CAD build for the part. Positions are in the model's coordinates, mm. Give positions to 0.01 mm unless a question says otherwise; leave off trailing zeros. Write each loop counter-clockwise with the first axis right and the second up, starting at its lowest first coordinate (ties: lowest second). Pieces come first, ordered by that corner, then holes. Notation, with made-up numbers: (25.5, 69.25) -> (53.5, 69.25) arc R20 cw to (53.5, 90.25) -> close; hole circle Ø4 at (88.5, -39). An arc over 180 degrees is marked (long way). Use one line per item in the form item = value. Start each with the question number.
from build123d import *

# Parameters (mm, degrees)
PAD017_DEPTH    = 1
PAD018_DEPTH    = 2
SKETCH041_R     = 3.5
PAD019_DEPTH    = 3.3
SKETCH042_R     = 2.55
POCKET018_DEPTH = 4.3
SKETCH043_R     = 2.8
PAD020_DEPTH    = 1.5
SKETCH044_R     = 2.1
POCKET019_DEPTH = 3
SKETCH045_R     = 3.5
PAD021_DEPTH    = 5.8
SKETCH046_R     = 2.55
POCKET020_DEPTH = 3.8
SKETCH047_R     = 2.6
POCKET021_DEPTH = 1.7
POCKET025_DEPTH = 2


with BuildPart() as part:
    # Sketch038 → Pad017 (new body)
    with BuildSketch(Plane.XZ):
        with BuildLine():
            ThreePointArc((6, 16), (8.928932, 8.928932), (16, 6))
            Line((16, 6), (185.51, 6))
            ThreePointArc((185.51, 6), (192.581068, 8.928932), (195.51, 16))
            Line((195.51, 16), (195.51, 107.04))
            ThreePointArc((195.51, 107.04), (192.581068, 114.111068), (185.51, 117.04))
            Line((185.51, 117.04), (96.718237, 117.04))
            ThreePointArc((96.718237, 117.04), (95.677689, 117.177713), (94.70879, 117.58137))
            Line((94.70879, 117.58137), (67.290497, 133.511257))
            ThreePointArc((67.290497, 133.511257), (65.837149, 134.116742), (64.276328, 134.323311))
            Line((64.276328, 134.323311), (41.441667, 134.323311))
            ThreePointArc((41.441667, 134.323311), (36.445319, 132.985672), (32.785632, 129.330611))
            Line((32.785632, 129.330611), (9.11531, 88.412125))
            ThreePointArc((9.11531, 88.412125), (6.792371, 82.814067), (6, 76.805203))
            Line((6, 76.805203), (6, 16))
        make_face()
    extrude(amount=PAD017_DEPTH)

    # Sketch040 (on Face15 of Pad017) → Pad018 (join)
    with BuildSketch(Plane(origin=(0, 0, 0), x_dir=(1, 0, 0), z_dir=(0, 1, 0))):
        with BuildLine():
            Line((16.1, -9.1), (185.41, -9.1))
            ThreePointArc((192.41, -16.1), (190.359747, -11.150253), (185.41, -9.1))
            Line((192.41, -16.1), (192.41, -106.94))
            ThreePointArc((185.41, -113.94), (190.359747, -111.889747), (192.41, -106.94))
            Line((185.41, -113.94), (95.883059, -113.94))
            ThreePointArc((95.883059, -113.94), (94.842511, -114.077713), (93.873612, -114.48137))
            Line((93.873612, -114.48137), (66.455319, -130.411257))
            ThreePointArc((63.44115, -131.223311), (65.001971, -131.016742), (66.455319, -130.411257))
            Line((63.44115, -131.223311), (41.499346, -131.223311))
            ThreePointArc((35.440122, -127.728421), (38.001902, -130.286964), (41.499346, -131.223311))
            Line((35.440122, -127.728421), (12.21531, -87.580081))
            ThreePointArc((9.1, -75.97316), (9.892371, -81.982024), (12.21531, -87.580081))
            Line((9.1, -75.97316), (9.1, -16.1))
            ThreePointArc((16.1, -9.1), (11.150253, -11.150253), (9.1, -16.1))
        make_face()
    extrude(amount=PAD018_DEPTH)

    # Sketch041 (on Face31 of Pad018) → Pad019 (join)
    with BuildSketch(Plane(origin=(0, 2, 0), x_dir=(1, 0, 0), z_dir=(0, 1, 0))):
        with Locations((145.11, -12.99)):
            Circle(SKETCH041_R)
        with Locations((64.452126, -127.45504)):
            Circle(SKETCH041_R)
        with Locations((14.14, -13.51)):
            Circle(SKETCH041_R)
        with Locations((19.14, -90.503884)):
            Circle(SKETCH041_R)
        with Locations((105.9, -108.54)):
            Circle(SKETCH041_R)
        with Locations((74.12, -12.75)):
            Circle(SKETCH041_R)
    extrude(amount=PAD019_DEPTH)

    # Sketch042 (on Face38 of Pad019) → Pocket018 (cut)
    with BuildSketch(Plane(origin=(0, 5.3, 0), x_dir=(1, 0, 0), z_dir=(0, 1, 0))):
        with Locations((145.11, -12.99)):
            Circle(SKETCH042_R)
        with Locations((19.14, -90.503884)):
            Circle(SKETCH042_R)
        with Locations((64.452126, -127.45504)):
            Circle(SKETCH042_R)
        with Locations((105.9, -108.54)):
            Circle(SKETCH042_R)
        with Locations((14.14, -13.51)):
            Circle(SKETCH042_R)
        with Locations((74.12, -12.75)):
            Circle(SKETCH042_R)
    extrude(amount=-POCKET018_DEPTH, mode=Mode.SUBTRACT)

    # Sketch043 (on Face31 of Pocket018) → Pad020 (join)
    with BuildSketch(Plane(origin=(0, 2, 0), x_dir=(1, 0, 0), z_dir=(0, 1, 0))):
        with Locations((185.580566, -111.078545)):
            Circle(SKETCH043_R)
    extrude(amount=PAD020_DEPTH)

    # Sketch044 (on Face45 of Pad020) → Pocket019 (cut)
    with BuildSketch(Plane(origin=(0, 3.5, 0), x_dir=(1, 0, 0), z_dir=(0, 1, 0))):
        with Locations((185.580566, -111.078545)):
            Circle(SKETCH044_R)
    extrude(amount=-POCKET019_DEPTH, mode=Mode.SUBTRACT)

    # Sketch045 (on Face31 of Pocket019) → Pad021 (join)
    with BuildSketch(Plane(origin=(0, 2, 0), x_dir=(1, 0, 0), z_dir=(0, 1, 0))):
        with Locations((188.21, -14.18)):
            Circle(SKETCH045_R)
    extrude(amount=PAD021_DEPTH)

    # Sketch046 (on Face45 of Pad021) → Pocket020 (cut)
    with BuildSketch(Plane(origin=(0, 7.8, 0), x_dir=(1, 0, 0), z_dir=(0, 1, 0))):
        with Locations((188.21, -14.18)):
            Circle(SKETCH046_R)
    extrude(amount=-POCKET020_DEPTH, mode=Mode.SUBTRACT)

    # Sketch047 (on Face5 of Pocket020) → Pocket021 (cut)
    with BuildSketch(Plane.XZ.offset(1)):
        with Locations((187.41, 103.94)):
            Circle(SKETCH047_R)
        with Locations((40.34577, 126.223311)):
            Circle(SKETCH047_R)
        with Locations((14.1, 77.580081)):
            Circle(SKETCH047_R)
        with Locations((103.873612, 14.1)):
            Circle(SKETCH047_R)
        with Locations((187.41, 19.1)):
            Circle(SKETCH047_R)
        with Locations((120.883059, 108.94)):
            Circle(SKETCH047_R)
        with Locations((19.1, 14.1)):
            Circle(SKETCH047_R)
    extrude(amount=-POCKET021_DEPTH, mode=Mode.SUBTRACT)

    # Sketch056 (on Face38 of Pocket021) → Pocket025 (cut)
    with BuildSketch(Plane(origin=(0, 2, 0), x_dir=(1, 0, 0), z_dir=(0, 1, 0))):
        Polygon((146.906174, -8.786863), (146.906174, -9.81445), (150.102356, -9.81445), (150.102356, -15.780038), (161.659576, -15.780038), (161.659576, -9.891122), (164.762894, -9.891122), (164.762894, -8.786863), align=None)
    extrude(amount=-POCKET025_DEPTH, mode=Mode.SUBTRACT)


with BuildPart() as part_1:
    # Body004 placement: moved
    add(part.part.moved(Location((0, -118.5, 0))))


solid = part_1.part
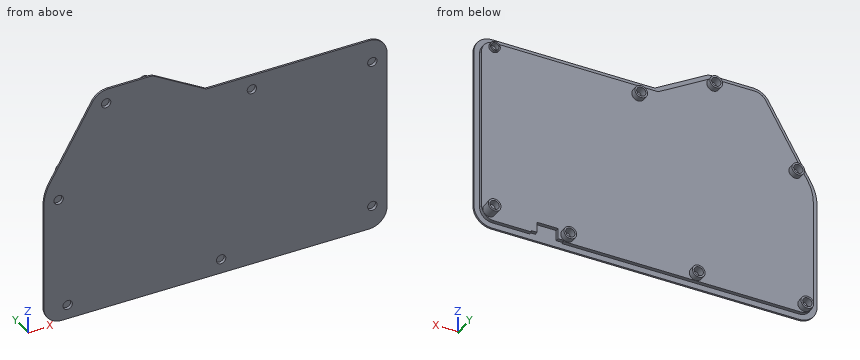
1) Pin check, flat tips, straight feed: pin 1 (4 mm diameter, centred on x = 102.5, z = 14, fed in from -Y); pin 2 (3 mm diameter, centred on x = 171.5, y = -118, fed in from +Z); pin 3 (12 mm diameter, centred on x = 175, z = 77, fed in from +Y); pin 4 (2 mm diameter, centred on x = 143.5, z = 12, fed in from +Y). Stop position of each tip, or through.
2) Cut at C-C (x = 74.12). Give the cut face in (y, z).
3) Cut at A-A (x = 177). Give the cut face in (y, z).
4) Wall check: line 1 along Z through (x, y) = (145, -114.75); line 2 along Z through (x, y) = (105.9, -114.6); line 3 along Z through (x, y) = (165.5, -117). Give the ranges that are in metal, low to high. Write a range as from..to.
5) Cut at B-B (z = 39.5). Give the cut face in (x, y), and give its area (3 significant figures).
Final values:
q1.pin_1 = -119.5
q1.pin_2 = 117.04
q1.pin_3 = -116.5
q1.pin_4 = -113.2
q2.outline = (-119.5, 6) -> (-118.5, 6) -> (-118.5, 9.1) -> (-116.5, 9.1) -> (-116.5, 9.25) -> (-113.2, 9.25) -> (-113.2, 10.2) -> (-117.5, 10.2) -> (-117.5, 15.3) -> (-113.2, 15.3) -> (-113.2, 16.25) -> (-116.5, 16.25) -> (-116.5, 125.96) -> (-118.5, 125.96) -> (-118.5, 129.54) -> (-119.5, 129.54) -> close
q3.outline = (-119.5, 6) -> (-118.5, 6) -> (-118.5, 9.1) -> (-116.5, 9.1) -> (-116.5, 113.94) -> (-118.5, 113.94) -> (-118.5, 117.04) -> (-119.5, 117.04) -> close
q4.line_1 = 9.49..10.44, 15.54..16.49
q4.line_2 = 105.04..105.99, 111.09..112.04
q4.line_3 = 9.1..113.94
q5.outline = (6, -119.5) -> (195.51, -119.5) -> (195.51, -118.5) -> (192.41, -118.5) -> (192.41, -116.5) -> (9.1, -116.5) -> (9.1, -118.5) -> (6, -118.5) -> close
q5.area = 556 mm^2
